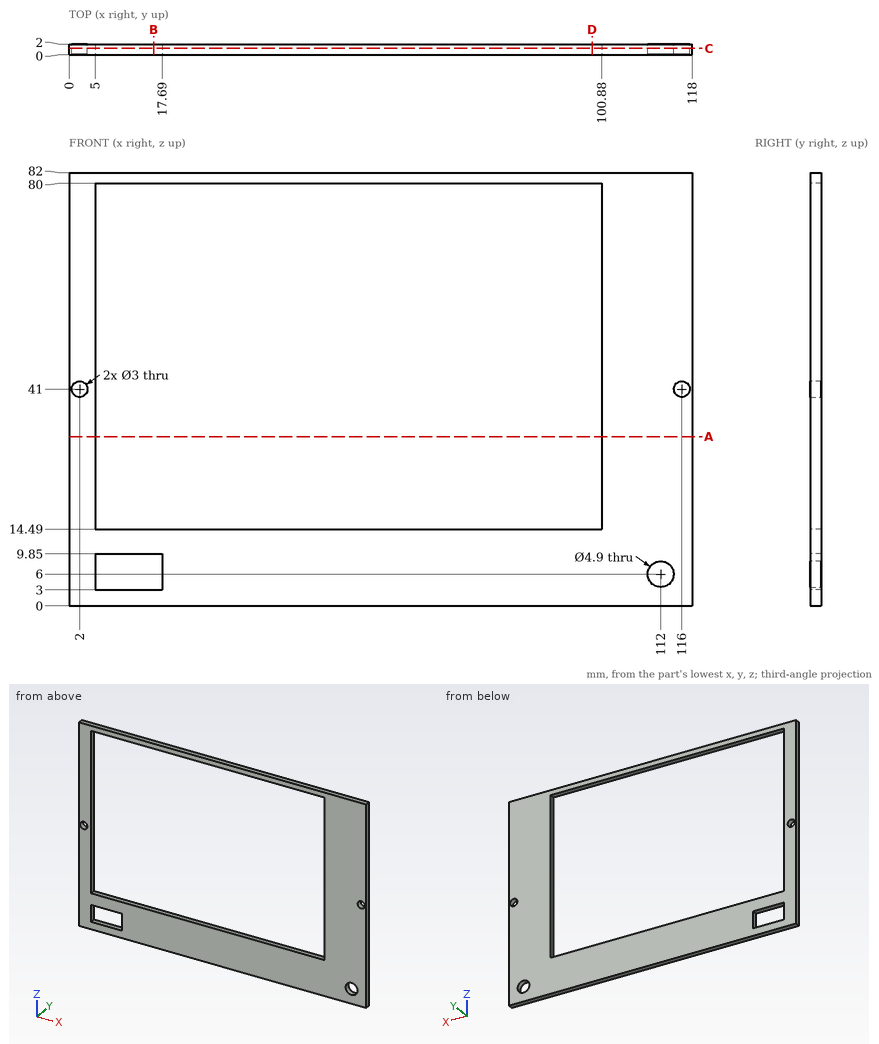
Geometry check sheet. Reference: drawing and pictorial views, mm from the part's lowest x, y, z. Round coordinates to 2 decimals unless told otherwise and drop trailing zeros. Order: outer loops, then holes, each group sorted by start corner. A loop starts at its lowest first (then second) coordinate and runs counter-clockwise, first axis right, second up. Notation, with made-up numbers: M 64,64.5 L 88,64.5 A11 cw 88,68.5 Z; hole C 63,77.25 d5. An arc over 180 degrees is marked long. One line per item, written item: value. Start each with the question number.
1. Scan lines: line 1 along Z through (x, y) = (9, 0.65); line 2 along X through (y, z) = (1.35, 43.5); line 3 along X through (y, z) = (1, 41). Record each from-to range of solid material in increasing order.
2. Section check B-B on x = 16. Enter the section's corners in (y, z), and give its area (3 significant figures).
3. Section check D-D on x = 99. Enter the section's corners in (y, z).
4. Gauge pin test, flat end, axial feed: P1, Ø4, axis at x = 112, z = 6, coming from the -Y side (3 decimals). Record the tip position at first contact, or that the pin passes through.
5. Section check A-A on z = 32. Enter the section's corners in (x, y).
6. Section check C-C on y = 1.15. Enter the section's corners in (x, z), and give its area (3 significant figures).
Results found:
1. line 1: 0 to 3, 9.85 to 14.49, 80 to 82
1. line 2: 0 to 5, 100.88 to 118
1. line 3: 0 to 0.5, 3.5 to 5, 100.88 to 114.5, 117.5 to 118
2. outline: M 0,0 L 2,0 L 2,3 L 0,3 Z; M 0,9.85 L 2,9.85 L 2,14.49 L 0,14.49 Z; M 0,80 L 2,80 L 2,82 L 0,82 Z
2. area: 19.3 mm^2
3. outline: M 0,0 L 2,0 L 2,14.49 L 0,14.49 Z; M 0,80 L 2,80 L 2,82 L 0,82 Z
4. P1: through
5. outline: M 0,0 L 5,0 L 5,2 L 0,2 Z; M 100.88,0 L 118,0 L 118,2 L 100.88,2 Z
6. outline: M 0,0 L 118,0 L 118,82 L 0,82 Z; hole C 2,41 d3; hole M 5,3 L 17.69,3 L 17.69,9.85 L 5,9.85 Z; hole M 5,14.49 L 100.88,14.49 L 100.88,80 L 5,80 Z; hole C 112,6 d4.9; hole C 116,41 d3
6. area: 3,270 mm^2
